For this review, use the dimensioned drawing (mm, ordinates from the lowest corner) and the shaded views. A direction names the side the tool comes from. Round coordinates to 2 decimals unless told otherwise and drop trailing zeros. Write each loop counter-clockwise with the first axis right and the second up, starting at its lowest first coordinate (ties: lowest second). Pieces come first, ordered by that corner, then holes.
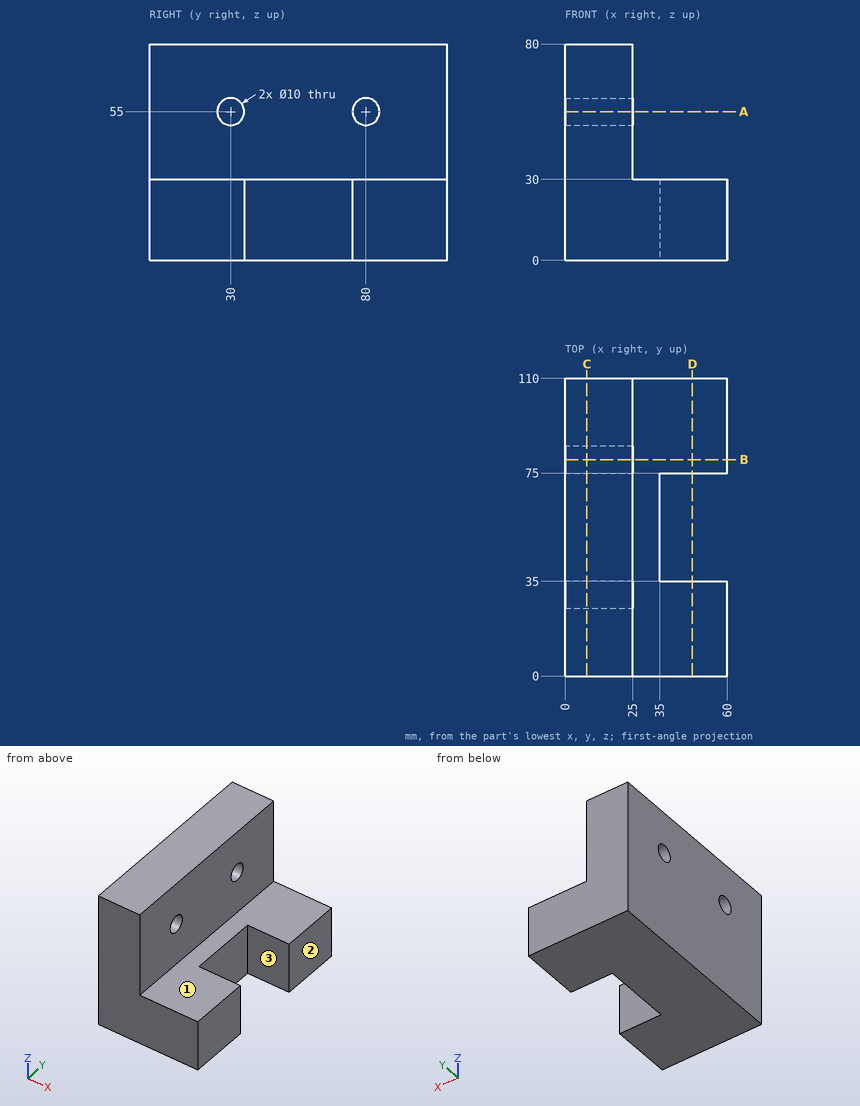
(1) We need section B-B, the plane y = 80. Give the boundary of the cut face in (x, z), and give its area (3 significant figures).
Geometry check:
outline: (0, 0) - (60, 0) - (60, 30) - (25, 30) - (25, 50) - (0, 50) - close; (0, 60) - (25, 60) - (25, 80) - (0, 80) - close
area: 2,800 mm2
(2) For the marked faces 1, 2 and 3, list the 3-axis set-ups (+Z, -Z, +X, -X, +Y, -Y) from which the entire face can be reached by the end or side of a thin tool; tool diameter is ignored.
Geometry check:
face 1: +Z, +X, +Y, -Y
face 2: +Z, -Z, +X, +Y, -Y
face 3: +Z, -Z, +X
(3) For line 1 along Z through (x, y) = (14.5, 30); line 2 along Y through (x, z) = (37.5, 18); line 3 along Z through (x, y) = (57, 86), list the stretches that pass through material, from the lowest coordinate up.
Geometry check:
line 1: z = 0 to 50, 60 to 80
line 2: y = 0 to 35, 75 to 110
line 3: z = 0 to 30
(4) We need section D-D, the plane x = 47. Give the boundary of the cut face in (y, z).
Geometry check:
outline: (0, 0) - (35, 0) - (35, 30) - (0, 30) - close; (75, 0) - (110, 0) - (110, 30) - (75, 30) - close
(5) For pin 1 Ø4 at (x, y) = (48.5, 27.5) entering from +Z; pin 2 Ø9 at (y, z) = (62.5, 15) entering from +X; pin 3 Ø11.5 at (y, z) = (30, 55) entering from +X, all flat-tipped, find the tip position at first contact; note any pin that passes through.
Geometry check:
pin 1: stops at z = 30
pin 2: stops at x = 35
pin 3: stops at x = 25
(6) We need section A-A, the plane z = 55. Give the boundary of the cut face in (x, y), and give its area (3 significant figures).
Geometry check:
outline: (0, 0) - (25, 0) - (25, 25) - (0, 25) - close; (0, 35) - (25, 35) - (25, 75) - (0, 75) - close; (0, 85) - (25, 85) - (25, 110) - (0, 110) - close
area: 2,250 mm2
(7) We need section C-C, the plane x = 8. Give the boundary of the cut face in (y, z).
Geometry check:
outline: (0, 0) - (110, 0) - (110, 80) - (0, 80) - close; hole circle Ø10 at (30, 55); hole circle Ø10 at (80, 55)
